Can you work these out from the drawing? Everything is in mm from the part's minimum corner. A direction names the side the tool comes from. Coordinates: 2 decimals unless noted, no trailing zeros. Write each loop counter-clockwise with the first axis right and the second up, starting at its lowest first coordinate (ties: lowest second). Pieces come first, ordered by that corner, then holes. Notation, with made-up numbers: M 80.25,44 L 95.25,44 A20 ccw 95.25,76 Z; hole C 63,26 d11. An arc over 180 degrees is marked long. Answer as a JSON object with one key per item and string values. Group by question number.
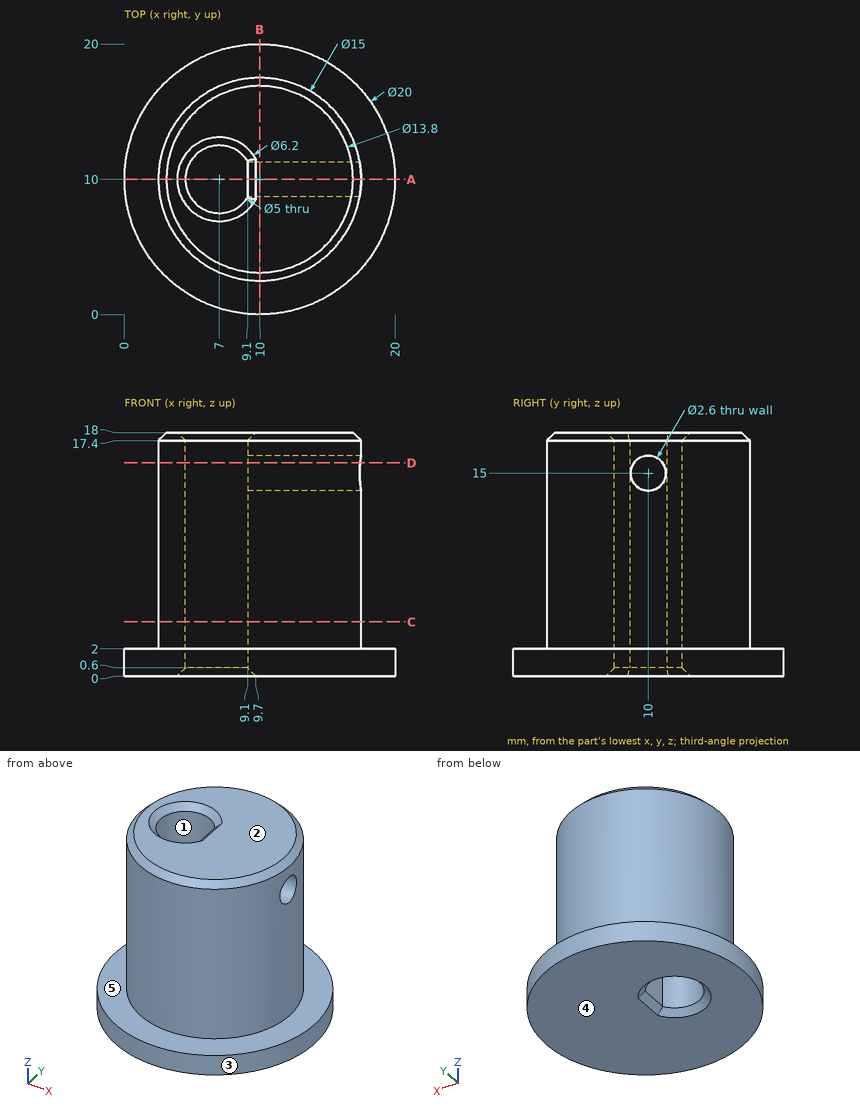
Q1. We'd pull the mould along X, two halves only. Please class the marked faces 1, 2 and 3: pulls with the +X half, pulls with the -X half, needs draft (parallel to the pull), parting line crosses it, or undercut.
Q2. If we section it at B-B on x = 10: List the corners of the cut face in (y, z) for me, and give its area (3 significant figures).
Q3. Please list where these lines run through material, in increasing order: L1, parallel to Z at x = 15.5, y = 10; L2, parallel to Y at x = 7, z = 5; L3, parallel to Z at x = 16.75, y = 16.
Q4. If we section it at A-A on y = 10: List the corners of the cut face in (x, z) for me, and give its area (3 significant figures).
Q5. If we section it at D-D on z = 15.75: List the corners of the cut face in (x, y) for me, and give its area (3 significant figures).
Q6. If we section it at C-C on z = 4: List the corners of the cut face in (x, y) for me.
Q7. Will these pins go through, and if not, where does the flat tip stop? pin 1 (4.5 mm diameter, centred on x = 7, y = 10, fed in from -Z); pin 2 (3.5 mm diameter, centred on y = 10, z = 15, fed in from -X); pin 3 (3 mm diameter, centred on y = 7.5, z = 7.5, fed in from -X).
Q8. On a 3-axis mill with a long thin cutter (end or side, diameter ignored), from which of +Z, -Z, +X, -X, +Y, -Y can I reach the whole of each face in a straight line? I mean the marked faces 4 and 5. Say none if no direction works.
Reply:
{
 "1": {"face 1": "undercut", "face 2": "needs draft", "face 3": "parting line crosses it"},
 "2": {"outline": "M 0,0 L 20,0 L 20,2 L 17.5,2 L 17.5,17.4 L 16.9,18 L 3.1,18 L 2.5,17.4 L 2.5,2 L 0,2 Z; hole C 10,15 d2.6", "area": "274 mm^2"},
 "3": {"L1": "0 to 13.7, 16.3 to 18", "L2": "3.13 to 7.5, 12.5 to 16.87", "L3": "0 to 2"},
 "4": {"outline": "M 0,0 L 3.9,0 L 4.5,0.6 L 4.5,17.4 L 3.9,18 L 3.1,18 L 2.5,17.4 L 2.5,2 L 0,2 Z; M 9.1,0.6 L 9.7,0 L 20,0 L 20,2 L 17.5,2 L 17.5,13.7 L 9.1,13.7 Z; M 9.1,16.3 L 17.5,16.3 L 17.5,17.4 L 16.9,18 L 9.7,18 L 9.1,17.4 Z", "area": "174 mm^2"},
 "5": {"outline": "M 9.1,8.64 A2.5 cw long 9.1,11.36 L 9.1,11.06 L 17.42,11.06 A7.5 ccw long 17.42,8.94 L 9.1,8.94 Z", "area": "140 mm^2"},
 "6": {"outline": "C 10,10 d15; hole M 9.1,8.64 L 9.1,11.36 A2.5 ccw long Z"},
 "7": {"pin 1": "z = 0.45", "pin 2": "x = 2.5", "pin 3": "x = 2.57"},
 "8": {"face 4": "-Z, +X, -X, +Y, -Y", "face 5": "+Z"}
}
